Design review of the part shown in the three views and the two pictorial views. Dimensions are in mm from the part's minimum x, y and z. A direction names the side the tool comes from. Round coordinates to 2 decimals unless told otherwise and drop trailing zeros. Order: outer loops, then holes, each group sorted by start corner. A loop starts at its lowest first (then second) coordinate and runs counter-clockwise, first axis right, second up. Notation, with made-up numbers: M -15.5,39.5 L -10.5,39.5 A17 cw -10.5,46.5 Z; hole C -31.75,-13 d1. An arc over 180 degrees is marked long. Use a Markdown table: item, result. Add a question column.
(1) Take a section at B-B (x = 50). Write out the cut boundary in (y, z), then the cut area to 3 significant figures.
(2) Take a section at D-D (z = 28.5). Write out the cut boundary in (x, y), then the cut area to 3 significant figures.
(3) To check wall thickness, follow probe 1 along X at (y, z) = (13.5, 60); probe 2 along X at (y, z) = (4.5, 58); probe 3 along Y at (x, z) = (17.5, 102). State the ranges of each line that lie inside material, in increasing order. Write a range as from..to.
(4) For pin 1 (1.5 mm diameter, centred on y = 11.5, z = 32.5, fed in from -X); pin 2 (1 mm diameter, centred on y = 13, z = 33.5, fed in from +X); pin 3 (5 mm diameter, centred on x = 75, y = 11, fed in from -Z), all flat-tipped, find the tip position at first contact; note any pin that passes through.
(5) Take a section at C-C (y = 13.5). Write out the cut boundary in (x, z).
(6) Take a section at A-A (z = 45). Write out the cut boundary in (x, y).
(7) Machinability: for the marked faces 1 and 2, which of the approach directions +Z, -Z, +X, -X, +Y, -Y give a long, thin tool a straight path to every point of the face, cutting with its end or side? Answer none if there is none.
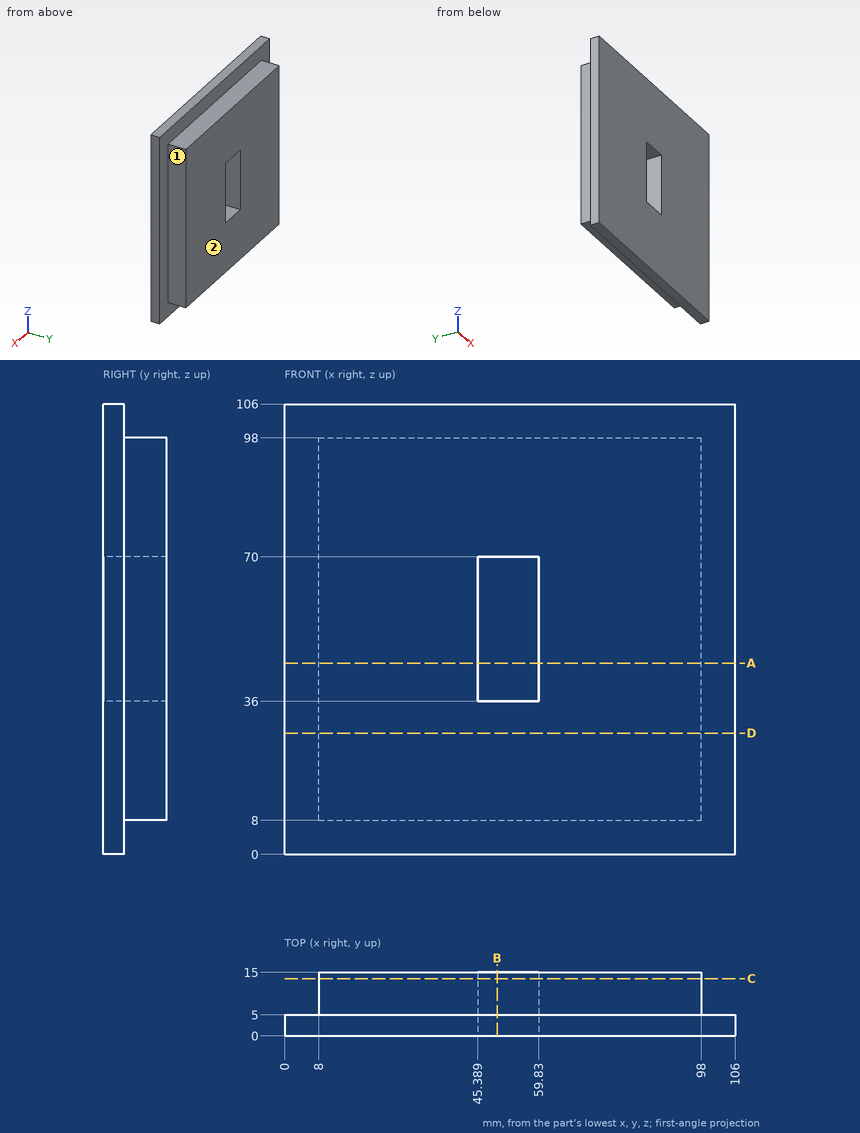
Verdict:
| question | item | result |
|---|---|---|
| 1 | outline | M 0,0 L 5,0 L 5,8 L 15,8 L 15,36 L 0,36 Z; M 0,70 L 15,70 L 15,98 L 5,98 L 5,106 L 0,106 Z |
| 1 | area | 920 mm^2 |
| 2 | outline | M 0,0 L 106,0 L 106,5 L 98,5 L 98,15 L 8,15 L 8,5 L 0,5 Z |
| 2 | area | 1,430 mm^2 |
| 3 | probe 1 | x = 8..45.39, 59.83..98 |
| 3 | probe 2 | x = 0..45.39, 59.83..106 |
| 3 | probe 3 | y = 0..5 |
| 4 | pin 1 | stops at x = 8 |
| 4 | pin 2 | stops at x = 98 |
| 4 | pin 3 | stops at z = 8 |
| 5 | outline | M 8,8 L 98,8 L 98,98 L 8,98 Z; hole M 45.39,36 L 59.83,36 L 59.83,70 L 45.39,70 Z |
| 6 | outline | M 0,0 L 45.39,0 L 45.39,15 L 8,15 L 8,5 L 0,5 Z; M 59.83,0 L 106,0 L 106,5 L 98,5 L 98,15 L 59.83,15 Z |
| 7 | face 1 | +Z, -Z, +X, +Y |
| 7 | face 2 | +Z, -Z, +X, -X, +Y |
